Check sheet for the modelled part. Datum: model origin and axes. Units: mm. A direction names the side the tool comes from. Round coordinates to 2 decimals unless told otherwise and drop trailing zeros. Order: outer loops, then holes, each group sorted by start corner. A loop starts at its lowest first (then second) coordinate and runs counter-clockwise, first axis right, second up. Notation, with made-up numbers: (77.25, -3) -> (119.25, -3) arc R15 cw to (119.25, 3) -> close; hole circle Ø8 at (60, 67). An arc over 180 degrees is marked (long way). Answer in a Markdown table with one row per item. Add a question column.
1. Sectioned sample at A-A, the plane z = 551.5. Record the boundary of the cut face in (x, y), then the cut area to 3 significant figures.
2. Draft check along Z on faces 1 (the cylindrical face through (30.5, 12.6, 597)), 2 (the flat face through (0, 4, 558)), 3 (the flat face through (-9, -9, 0)). Enter one of: +Z half, -Z half, draft (parallel to the pull), parting line (faces both ways), or undercut.
3. Access from +Z, -Z, +X, -X, +Y, -Y to the whole of each face (thin tool, end or side, straight path). Record for faces 4 (the flat face through (3.4, -0.1, 58)), 5 (the flat face through (-1, -1, 631)), 6 (the cylindrical face through (-4.336, 19.524, 16.731)).
4. Material ranges on L1, parallel to X at y = 0, z = 21; L2, parallel to Z at x = -23, y = -8.5, recorded low to high. Write a range as from..to.
5. Depth check by flat-ended pin: P1, Ø6, axis at y = 5, z = 326.5, coming from the -X side. Enter the tip coordinate at first touch or a pass-through.
```python
from build123d import *


with BuildPart() as f1:
    # F0 (on Front) → F1 (revolve)
    with BuildSketch(Plane.XZ):
        with BuildLine():
            Line((0, 631), (0, 32))
            Line((0, 32), (12.5, 32))
            Line((12.5, 32), (12.5, 0))
            Line((12.5, 0), (20, 0))
            Line((20, 0), (20, 33))
            Line((20, 33), (28, 33))
            Line((28, 33), (28, 41))
            ThreePointArc((28, 41), (15.589403, 46.664003), (8, 58))
            Line((8, 58), (3, 58))
            Line((3, 58), (3, 558))
            Line((3, 558), (18, 558))
            ThreePointArc((18, 558), (28.606602, 562.393398), (33, 573))
            Line((33, 573), (33, 620.287857))
            ThreePointArc((33, 620.287857), (34.170683, 626.097332), (37.5, 631))
            Line((37.5, 631), (0, 631))
        make_face()
    revolve(axis=Axis((0, 0, 331.5), (0, 0, -1)))


solid = f1.part
```
Answer key:
| question | item | result |
|---|---|---|
| 1 | outline | circle Ø6 at (0, 0) |
| 1 | area | 28.3 mm² |
| 2 | face 1 | draft |
| 2 | face 2 | undercut |
| 2 | face 3 | -Z half |
| 3 | face 4 | none |
| 3 | face 5 | +Z, +X, -X, +Y, -Y |
| 3 | face 6 | -Z |
| 4 | L1 | x = -20..-12.5, 12.5..20 |
| 4 | L2 | z = 33..41.79, 559.49..631 |
| 5 | P1 | stops at x = -2.24 |
